```python
from build123d import *


with BuildPart() as part:
    # Sketch 1 → Revolve 1 (revolve)
    with BuildSketch(Plane.XY, mode=Mode.PRIVATE) as revolve_1_sk:
        with BuildLine():
            Line((-11, 0), (-11, 5))
            Line((-11, 5), (-10, 6))
            Line((-10, 6), (-8, 6))
            Line((-8, 6), (-8, 9))
            Line((-8, 9), (-9, 10))
            Line((-9, 10), (-9, 15))
            ThreePointArc((-9, 15), (-7.535533906, 18.535533906), (-4, 20))
            Line((-4, 20), (4, 20))
            ThreePointArc((4, 20), (7.535533906, 18.535533906), (9, 15))
            Line((9, 15), (9, 10))
            Line((9, 10), (8, 9))
            Line((8, 9), (8, 6))
            Line((8, 6), (10, 6))
            Line((10, 6), (11, 5))
            Line((11, 5), (11, 0))
            Line((11, 0), (-11, 0))
        make_face()
    revolve(revolve_1_sk.sketch.rotate(Axis((11, 0, 0), (-1, 0, 0)), 270), axis=Axis((11, 0, 0), (-1, 0, 0)))


solid = part.part
```
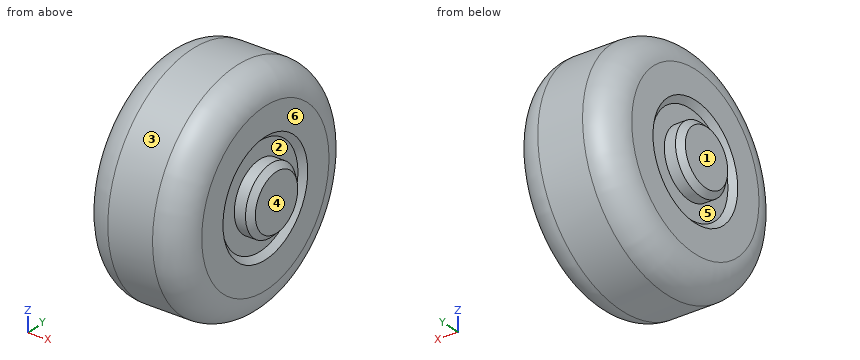
Model file for the job. Use its own axes, mm. Face numbers are marked on the shaded views. A direction names the side the tool comes from. Coordinates: 2 decimals unless noted, no trailing zeros. Write each loop counter-clockwise with the first axis right and the second up, starting at its lowest first coordinate (ties: lowest second). Pieces come first, ordered by that corner, then holes. Notation, with made-up numbers: (-16, 21) - (-2, 21) arc R18 ccw to (-2, 41) - close; hole circle Ø7 at (-26, 51.5). An arc over 180 degrees is marked (long way). Use a Markdown table: item, result. Add a question column.
Item 1: Drill centre lines: line 1 along X through (y, z) = (12, -8); line 2 along X through (y, z) = (-3, -7); line 3 along Y through (x, z) = (-6, 14). Where is each one in solid material? Low to high.
Item 2: Band-saw the part on A-A, the plane y = 0. Write the cut outline in (x, z), and give its area (3 significant figures).
Item 3: Band-saw the part on C-C, the plane x = 1.5. Write the cut outline in (y, z).
Item 4: Two-plate mould, pull along Y, no slides. Class the marked faces 1, 2 and 3: pulls with the +Y half, pulls with the -Y half, needs draft (parallel to the pull), parting line crosses it, or undercut.
Item 5: 3-axis set-ups, long thin cutter, end or side, ignore diameter. For the marked faces 4, 5 and 6: which of +Z, -Z, +X, -X, +Y, -Y reach the whole face in a straight line?
Item 6: Drop flat-ended pins along their axis: pin 1 (10 mm diameter, centred on x = -6, y = -11.5, fed in from +Z); pin 2 (12 mm diameter, centred on y = -16, z = 1, fed in from -X); pin 3 (6 mm diameter, centred on y = -12.5, z = -16, fed in from +X). Give the stop position or say it passes through.
A:
| question | item | result |
|---|---|---|
| 1 | line 1 | x = -9 to 9 |
| 1 | line 2 | x = -8 to 8 |
| 1 | line 3 | y = -13.69 to 13.69 |
| 2 | outline | (-11, -5) - (-10, -6) - (-8, -6) - (-8, -9) - (-9, -10) - (-9, -15) arc R5 ccw to (-4, -20) - (4, -20) arc R5 ccw to (9, -15) - (9, -10) - (8, -9) - (8, -6) - (10, -6) - (11, -5) - (11, 5) - (10, 6) - (8, 6) - (8, 9) - (9, 10) - (9, 15) arc R5 ccw to (4, 20) - (-4, 20) arc R5 ccw to (-9, 15) - (-9, 10) - (-8, 9) - (-8, 6) - (-10, 6) - (-11, 5) - close |
| 2 | area | 731 mm² |
| 3 | outline | circle Ø40 at (0, 0) |
| 4 | face 1 | needs draft |
| 4 | face 2 | undercut |
| 4 | face 3 | parting line crosses it |
| 5 | face 4 | +Z, -Z, +X, +Y, -Y |
| 5 | face 5 | -X |
| 5 | face 6 | +X |
| 6 | pin 1 | stops at z = 18.81 |
| 6 | pin 2 | stops at x = -9 |
| 6 | pin 3 | stops at x = 8.44 |
